Model file for the job. Use its own axes, mm. A direction names the side the tool comes from. Round coordinates to 2 decimals unless told otherwise and drop trailing zeros. Order: outer loops, then holes, each group sorted by start corner. A loop starts at its lowest first (then second) coordinate and runs counter-clockwise, first axis right, second up. Notation, with made-up numbers: M -4.75,26 L 12.25,26 A19 cw 12.25,55 Z; hole C -2,19.25 d5. An arc over 180 degrees is marked long. Return JSON: item names as keys, results as strings. Group by question number.
Item 1: Probe line 1 along Y through (x, z) = (41, 15); line 2 along Z through (x, y) = (39, 0.5); line 3 along Z through (x, y) = (86.5, -6.5). List the from-to ranges inside material, lowest first.
Item 2: Which spindle directions (+Z, -Z, +X, -X, +Y, -Y) get a long thin tool onto all of the face, cutting with end or side? Do faces 1 (the face through (49, -2.5, 59)), 2 (the face through (0, 0, 52)), 3 (the face through (49, 2.5, 58)). Say none if no direction does.
Item 3: Slice it at C-C on z = 72. Write the cut outline in (x, y), then the cut area to 3 significant figures.
Item 4: Pin check, flat tips, straight feed: pin 1 Ø1 at (x, y) = (77, 4.5) entering from -Z; pin 2 Ø5 at (x, z) = (42, 27) entering from -Y; pin 3 Ø3 at (x, z) = (71, 12) entering from +Y. Stop position of each tip, or through.
Item 5: Slice it at B-B on y = -4.5. Write the cut outline in (x, z), then the cut area to 3 significant figures.
Item 6: Slice it at A-A on x = 82. Write the cut outline in (y, z).
from build123d import *

# Parameters (mm, degrees)
BOSS_EXTRUDE1_DEPTH = 100


with BuildPart() as part:
    # Sketch1 → Boss-Extrude1 (new body)
    with BuildSketch(Plane(origin=(0, 0, 0), x_dir=(0, 0, -1), z_dir=(1, 0, 0))):
        with BuildLine():
            ThreePointArc((0, -2.5), (-2.5, 0), (0, 2.5))
            Line((0, 2.5), (-7.071067812, 2.5))
            ThreePointArc((-7.071067812, 2.5), (-7.5, 0), (-7.071067812, -2.5))
            Line((-7.071067812, -2.5), (0, -2.5))
        make_face()
        with BuildLine():
            Line((-7.071067812, 2.5), (0, 2.5))
            ThreePointArc((0, 2.5), (1.767766953, 1.767766953), (2.5, 0))
            ThreePointArc((2.5, 0), (1.767766953, -1.767766953), (0, -2.5))
            Line((0, -2.5), (-7.071067812, -2.5))
            ThreePointArc((-7.071067812, -2.5), (1.26826484, -7.391989197), (7.5, 0))
            ThreePointArc((7.5, 0), (1.26826484, 7.391989197), (-7.071067812, 2.5))
        make_face()
        with BuildLine():
            ThreePointArc((-7.071067812, -2.5), (-7.5, 0), (-7.071067812, 2.5))
            Line((-7.071067812, 2.5), (-110, 2.5))
            Line((-110, 2.5), (-110, -2.5))
            Line((-110, -2.5), (-7.071067812, -2.5))
        make_face()
    extrude(amount=BOSS_EXTRUDE1_DEPTH)


solid = part.part
Output values:
{
 "1": {"line 1": "-2.5 to 2.5", "line 2": "-7.48 to -2.45, 2.45 to 110", "line 3": "-3.74 to 3.74"},
 "2": {"face 1": "+Z, +X, -X, -Y", "face 2": "+Z, -Z, -X, +Y, -Y", "face 3": "+Z, +X, -X, +Y"},
 "3": {"outline": "M 0,-2.5 L 100,-2.5 L 100,2.5 L 0,2.5 Z", "area": "500 mm²"},
 "4": {"pin 1": "z = -6.34", "pin 2": "y = -2.5", "pin 3": "y = 2.5"},
 "5": {"outline": "M 0,-6 L 100,-6 L 100,6 L 0,6 Z", "area": "1,200 mm²"},
 "6": {"outline": "M -2.5,7.07 A7.5 ccw long 2.5,7.07 L 2.5,110 L -2.5,110 Z; hole C 0,0 d5"}
}
